Design review of the part built by this model. Coordinates are the model's own, in mm. Coordinates: 2 decimals unless noted, no trailing zeros. Order: outer loops, then holes, each group sorted by start corner. A loop starts at its lowest first (then second) coordinate and runs counter-clockwise, first axis right, second up. Notation, with made-up numbers: (83, 18) - (107, 18) arc R35 cw to (107, 56) - close; hole circle Ø1 at (25, 50.25). An arc over 180 degrees is marked (long way). Write each question's results on one line, items separated by ' | '. Start each with the question number.
```python
from build123d import *

# Parameters (mm, degrees)
SKETCH1_W                              = 14
SKETCH1_H                              = 12
SKETCH2_R                              = 3.3
SKETCH2_R_2                            = 3
CUT_8XTIE_D6_6_2XDOWEL_D6_PCD128_DEPTH = 150


with BuildPart() as part:
    # Sketch1 → REV_Interstage_Spacer (revolve)
    with BuildSketch(Plane(origin=(0, 0, 0), x_dir=(1, 0, 0), z_dir=(0, 1, 0))):
        with Locations((63, 13.5)):
            Rectangle(SKETCH1_W, SKETCH1_H)
    revolve(axis=Axis((0, 0, 150), (0, 0, -1)))

    # Sketch2 → CUT_8xTie_D6.6_2xDowel_D6_PCD128 (cut, symmetric)
    with BuildSketch(Plane.XY):
        with Locations(Location((64, 0, 0), (0, 0, 180))):
            Circle(SKETCH2_R)
        with Locations(Location((45.2548, 45.2548, 0), (0, 0, 180))):
            Circle(SKETCH2_R)
        with Locations(Location((0, 64, 0), (0, 0, 180))):
            Circle(SKETCH2_R)
        with Locations(Location((-45.2548, 45.2548, 0), (0, 0, 180))):
            Circle(SKETCH2_R)
        with Locations(Location((-64, 0, 0), (0, 0, 180))):
            Circle(SKETCH2_R)
        with Locations(Location((-45.2548, -45.2548, 0), (0, 0, 180))):
            Circle(SKETCH2_R)
        with Locations(Location((0, -64, 0), (0, 0, 180))):
            Circle(SKETCH2_R)
        with Locations(Location((45.2548, -45.2548, 0), (0, 0, 180))):
            Circle(SKETCH2_R)
        with Locations(Location((24.4917, 59.1283, 0), (0, 0, 180))):
            Circle(SKETCH2_R_2)
        with Locations(Location((-24.4917, -59.1283, 0), (0, 0, 180))):
            Circle(SKETCH2_R_2)
    extrude(amount=CUT_8XTIE_D6_6_2XDOWEL_D6_PCD128_DEPTH, both=True, mode=Mode.SUBTRACT)


solid = part.part
```
(1) Mouldability with a two-part tool opening along Y and no side actions: class faces 1 (the face through (67.3, -0.1, -13.4)), 2 (the face through (21.1, -52.2, -19.5)), 3 (the face through (0.43, -67.27, -13.42)), 4 (the face through (-55.55, 42.594, -13.584)) as +Y half, -Y half, draft (parallel to the pull), parting line (faces both ways), or undercut.
(2) Clearance check with flat-ended pins moving along their axes: pin 1 (4 mm diameter, centred on y = -4.5, z = -8.5, fed in from +X); pin 2 (3 mm diameter, centred on x = 36.5, z = -11.5, fed in from -Y); pin 3 (6 mm diameter, centred on x = 14, z = -10.5, fed in from -Y). State where each tip first meets the part, or that it passes through.
(3) To check wall thickness, follow line 1 along Y through (x, z) = (0, -14.25); line 2 along X through (y, z) = (46.5, -17.5); line 3 along X through (y, z) = (37, -13.75). State the ranges of each line that lie inside material, in increasing order. Write a range as [from, to].
(4) Take a section at D-D (x = -25.5). State the section outline as (y, z) points, plus the area to 3 significant figures.
(5) Take a section at A-A (y = 0). State the section outline as (x, z) points.
(6) Take a section at C-C (y = -36). State the section outline as (x, z) points, plus the area to 3 significant figures.
Worked out:
1) face 1: undercut | face 2: draft | face 3: undercut | face 4: parting line
2) pin 1: x = 69.96 | pin 2: y = -60.62 | pin 3: y = -69.13
3) line 1: [-70, -67.3], [-60.7, -56], [56, 60.7], [67.3, 70] | line 2: [-52.32, -48.31], [-42.2, -31.2], [31.2, 42.2], [48.31, 52.32] | line 3: [-59.42, -42.04], [42.04, 59.42]
4) outline: (-65.19, -19.5) - (-61.95, -19.5) - (-61.95, -7.5) - (-65.19, -7.5) - close; (-56.3, -19.5) - (-49.86, -19.5) - (-49.86, -7.5) - (-56.3, -7.5) - close; (49.86, -19.5) - (65.19, -19.5) - (65.19, -7.5) - (49.86, -7.5) - close | area: 300 mm^2
5) outline: (-70, -19.5) - (-67.3, -19.5) - (-67.3, -7.5) - (-70, -7.5) - close; (-60.7, -19.5) - (-56, -19.5) - (-56, -7.5) - (-60.7, -7.5) - close; (56, -19.5) - (60.7, -19.5) - (60.7, -7.5) - (56, -7.5) - close; (67.3, -19.5) - (70, -19.5) - (70, -7.5) - (67.3, -7.5) - close
6) outline: (-60.03, -19.5) - (-42.9, -19.5) - (-42.9, -7.5) - (-60.03, -7.5) - close; (42.9, -19.5) - (60.03, -19.5) - (60.03, -7.5) - (42.9, -7.5) - close | area: 411 mm^2
